Model file for the job. Use its own axes, mm. A direction names the side the tool comes from. Give positions to 0.01 mm unless a question says otherwise; leave off trailing zeros. Loops run counter-clockwise (first coordinate to the right, second up) from the corner with the lowest first, then second, coordinate; pieces in that order, holes last. Notation, with made-up numbers: M 34.5,11.5 L 75.5,11.5 A10 ccw 75.5,24.5 Z; hole C 23,-33.75 d9. An arc over 180 degrees is marked long. Answer in a Markdown table with one row per item.
```python
from build123d import *

# Parameters (mm, degrees)
F1_DEPTH = 12.7
F2_D     = 6.35
F3_D     = 6.5278
F4_D     = 6.5278
F5_D     = 6.5278


with BuildPart() as f1:
    # F0 (on Front) → F1 (new body)
    with BuildSketch(Plane.XZ):
        with BuildLine():
            Line((0, 51.6978976429), (0, 70.7478976429))
            Line((0, 70.7478976429), (-101.6, 70.7478976429))
            Line((-101.6, 70.7478976429), (-101.6, 83.4478976429))
            Line((-101.6, 83.4478976429), (-152.4, 83.4478976429))
            Line((-152.4, 83.4478976429), (-152.4, 19.9478976429))
            Line((-152.4, 19.9478976429), (-25.4, -68.9521023571))
            Line((-25.4, -68.9521023571), (0, -68.9521023571))
            Line((0, -68.9521023571), (0, -46.7271023571))
            ThreePointArc((0, -46.7271023571), (-20.2055762724, -38.3576786296), (-28.575, -18.1521023571))
            ThreePointArc((-28.575, -18.1521023571), (-25.4, -14.9771023571), (-22.225, -18.1521023571))
            ThreePointArc((-22.225, -18.1521023571), (-15.7154482119, -33.867550569), (0, -40.3771023571))
            Line((0, -40.3771023571), (0, -18.1521023571))
            Line((0, -18.1521023571), (0, 51.6978976429))
        make_face()
        with BuildLine():
            Line((101.6, 70.7478976429), (0, 70.7478976429))
            Line((0, 70.7478976429), (0, 51.6978976429))
            Line((0, 51.6978976429), (0, -18.1521023571))
            Line((0, -18.1521023571), (0, -40.3771023571))
            ThreePointArc((0, -40.3771023571), (15.7154482119, -33.867550569), (22.225, -18.1521023571))
            ThreePointArc((22.225, -18.1521023571), (25.4, -14.9771023571), (28.575, -18.1521023571))
            ThreePointArc((28.575, -18.1521023571), (20.2055762724, -38.3576786296), (0, -46.7271023571))
            Line((0, -46.7271023571), (0, -68.9521023571))
            Line((0, -68.9521023571), (25.4, -68.9521023571))
            Line((25.4, -68.9521023571), (152.4, 19.9478976429))
            Line((152.4, 19.9478976429), (152.4, 83.4478976429))
            Line((152.4, 83.4478976429), (101.6, 83.4478976429))
            Line((101.6, 83.4478976429), (101.6, 70.7478976429))
        make_face()
    extrude(amount=F1_DEPTH)

    # F2 (through all)
    with Locations(Plane(origin=(0, 0, 0), x_dir=(1, 0, 0), z_dir=(0, 1, 0))):
        with Locations((44.45, -58.0478976429), (-44.45, -58.0478976429)):
            Hole(F2_D / 2)

    # F3 (through all)
    with Locations(Plane(origin=(0, 0, 0), x_dir=(1, 0, 0), z_dir=(0, 1, 0))):
        with Locations((-127, -58.0478976429)):
            Hole(F3_D / 2)

    # F4 (through all)
    with Locations(Plane(origin=(0, 0, 0), x_dir=(1, 0, 0), z_dir=(0, 1, 0))):
        with Locations((0, 18.1521023571)):
            Hole(F4_D / 2)

    # F5 (through all)
    with Locations(Plane(origin=(0, 0, 0), x_dir=(1, 0, 0), z_dir=(0, 1, 0))):
        with Locations((127, -58.0478976429)):
            Hole(F5_D / 2)


solid = f1.part
```
Q1. Probe probe 1 along X at (y, z) = (-7.25, -26); probe 2 along Z at (x, y) = (-44.45, -7); probe 3 along Z at (x, y) = (-2, -8.25). List the from-to ranges inside material, lowest first.
Reported:
| item | result |
|---|---|
| probe 1 | -86.76 to -27.48, -20.79 to 20.79, 27.48 to 86.76 |
| probe 2 | -55.62 to 54.87, 61.22 to 70.75 |
| probe 3 | -68.95 to -46.66, -40.29 to -20.73, -15.57 to 70.75 |
Q2. Mould opens along Z. For faces 4 (the face through (-2, 0, 25)), 5 (the face through (1, -6, 70.748)), 6 (the face through (0.708, -6.439, -14.966)) say: released by +Z, released by -Z, zero draft, split by the parting line, or undercut.
Reported:
| item | result |
|---|---|
| face 4 | zero draft |
| face 5 | released by +Z |
| face 6 | undercut |
Q3. Saw through at A-A (x = -14). Give the cut face in (y, z).
Reported:
| item | result |
|---|---|
| outline | M -12.7,-68.95 L 0,-68.95 L 0,-43.06 L -12.7,-43.06 Z; M -12.7,-35.41 L 0,-35.41 L 0,70.75 L -12.7,70.75 Z |
Q4. Saw through at B-B (y = -9.75). Give the cut face in (x, z) (3 decimals), and give its area (3 significant figures).
Reported:
| item | result |
|---|---|
| outline | M -152.4,19.948 L -25.4,-68.952 L 25.4,-68.952 L 152.4,19.948 L 152.4,83.448 L 101.6,83.448 L 101.6,70.748 L -101.6,70.748 L -101.6,83.448 L -152.4,83.448 Z; hole C -127,58.048 d6.528; hole C -44.45,58.048 d6.35; hole M -28.575,-18.152 A28.575 ccw 28.575,-18.152 A3.175 ccw 22.225,-18.152 A22.225 cw -22.225,-18.152 A3.175 ccw Z; hole C 0,-18.152 d6.528; hole C 44.45,58.048 d6.35; hole C 127,58.048 d6.528 |
| area | 31,900 mm² |
Q5. Saw through at D-D (x = -127). Give the cut face in (y, z), and give its area (3 significant figures).
Reported:
| item | result |
|---|---|
| outline | M -12.7,2.17 L 0,2.17 L 0,54.78 L -12.7,54.78 Z; M -12.7,61.31 L 0,61.31 L 0,83.45 L -12.7,83.45 Z |
| area | 949 mm² |
Q6. Saw through at C-C (z = -37.5). Give the cut face in (x, y).
Reported:
| item | result |
|---|---|
| outline | M -70.33,-12.7 L -21.03,-12.7 L -21.03,0 L -70.33,0 Z; M -10.94,-12.7 L 10.94,-12.7 L 10.94,0 L -10.94,0 Z; M 21.03,-12.7 L 70.33,-12.7 L 70.33,0 L 21.03,0 Z |
Q7. Drop flat-ended pins along their axis: pin 1 (10.5 mm diameter, centred on x = 127, z = 58.05, fed in from +Y); pin 2 (3 mm diameter, centred on x = -16, y = -10, fed in from +Z); pin 3 (1 mm diameter, centred on y = -4, z = -50, fed in from -X). Give the stop position or say it passes through.
Reported:
| item | result |
|---|---|
| pin 1 | y = 0 |
| pin 2 | z = 70.75 |
| pin 3 | x = -53.19 |
Q8. 3-axis set-ups, long thin cutter, end or side, ignore diameter. For faces 1 (the face through (-101.6, -6, 77)), 2 (the face through (-25.47, -6.261, -14.978)), 3 (the face through (-2, -12.7, 25)): which of +Z, -Z, +X, -X, +Y, -Y reach the whole face in a straight line?
Reported:
| item | result |
|---|---|
| face 1 | +Z, +Y, -Y |
| face 2 | +Y, -Y |
| face 3 | +Z, -Z, +X, -X, -Y |
